Read the model definition and answer for the solid it produces. Units are mm, in the model's axes. Give positions to 0.01 mm unless a question says otherwise; leave off trailing zeros. Loops run counter-clockwise (first coordinate to the right, second up) from the corner with the lowest first, then second, coordinate; pieces in that order, holes last. Notation, with made-up numbers: (-28.75, 44.25) - (-24.75, 44.25) arc R21 ccw to (-24.75, 63.25) - close; hole circle Ø9 at (-19, -31.75). An arc over 180 degrees is marked (long way). Write item = value, one per line.
```python
from build123d import *

# Parameters (mm, degrees)
SKETCH_W   = 40
SKETCH_H   = 40
SKETCH_R   = 18
SKETCH_R_2 = 2
PAD_DEPTH  = 10
FILLET_R   = 2


with BuildPart() as part:
    # Sketch → Pad (new body)
    with BuildSketch(Plane.XY):
        with Locations((20, 20)):
            Rectangle(SKETCH_W, SKETCH_H)
        with Locations((20, 20)):
            Circle(SKETCH_R, mode=Mode.SUBTRACT)
        with Locations((4, 36)):
            Circle(SKETCH_R_2, mode=Mode.SUBTRACT)
        with Locations((36, 36)):
            Circle(SKETCH_R_2, mode=Mode.SUBTRACT)
        with Locations((36, 4)):
            Circle(SKETCH_R_2, mode=Mode.SUBTRACT)
        with Locations((4, 4)):
            Circle(SKETCH_R_2, mode=Mode.SUBTRACT)
    extrude(amount=PAD_DEPTH)

    # Fillet
    fillet_edges = [part.edges().sort_by_distance(p)[0] for p in [
        (40, 0, 5),
        (0, 0, 5),
        (40, 40, 5),
        (0, 40, 5),
    ]]
    fillet(fillet_edges, radius=FILLET_R)


solid = part.part
```
1) A cutting plane is placed at A-A on y = 20. Determine the outline of the cut face in (x, z).
Output:
outline = (0, 0) - (2, 0) - (2, 10) - (0, 10) - close; (38, 0) - (40, 0) - (40, 10) - (38, 10) - close
2) A cutting plane is placed at D-D on y = 36. Determine the outline of the cut face in (x, z).
Output:
outline = (0, 0) - (2, 0) - (2, 10) - (0, 10) - close; (6, 0) - (11.75, 0) - (11.75, 10) - (6, 10) - close; (28.25, 0) - (34, 0) - (34, 10) - (28.25, 10) - close; (38, 0) - (40, 0) - (40, 10) - (38, 10) - close
3) A cutting plane is placed at C-C on z = 1.5. Determine the outline of the cut face in (x, y), then the cut area to 3 significant figures.
Output:
outline = (0, 2) arc R2 ccw to (2, 0) - (38, 0) arc R2 ccw to (40, 2) - (40, 38) arc R2 ccw to (38, 40) - (2, 40) arc R2 ccw to (0, 38) - close; hole circle Ø4 at (4, 4); hole circle Ø36 at (20, 20); hole circle Ø4 at (4, 36); hole circle Ø4 at (36, 4); hole circle Ø4 at (36, 36)
area = 528 mm²
4) The mould has two halves that part along Y. Classify faces 1 (the face through (2.4, 2.8, 4.9)), 2 (the face through (0, 20, 5)), 3 (the face through (39.4, 39.43, 5.07)): pulls with the +Y half, pulls with the -Y half, needs draft (parallel to the pull), parting line crosses it, or undercut.
Output:
face_1 = undercut
face_2 = needs draft
face_3 = pulls with the +Y half
5) Find the intervals of material crossed by probe 1 along Y at (x, z) = (36, 6.5); probe 2 along X at (y, z) = (20.5, 0.5); probe 3 along Y at (x, z) = (33.5, 9.5), in increasing order.
Output:
probe_1 = 0 to 2, 6 to 11.75, 28.25 to 34, 38 to 40
probe_2 = 0 to 2.01, 37.99 to 40
probe_3 = 0 to 8.09, 31.91 to 40
